CAD build for the part. Positions are in the model's coordinates, mm. A direction names the side the tool comes from. Coordinates: 2 decimals unless noted, no trailing zeros. Write each loop counter-clockwise with the first axis right and the second up, starting at its lowest first coordinate (ties: lowest second). Pieces come first, ordered by that corner, then holes. Notation, with made-up numbers: (-38, 12) - (-18, 12) arc R27 ccw to (-18, 28) - close; hole circle Ø3 at (31.25, 58). An arc over 180 degrees is marked (long way). Answer in a Markdown table with one row per item. Add a question column.
Q1. Two-plate mould, pull along Z, no slides. Class faces 1 (the flat face through (0, -15, 250)), 2 (the cylindrical face through (4.77, -10.61, 51.5)): +Z half, -Z half, draft (parallel to the pull), parting line (faces both ways), or undercut.
Q2. 3-axis set-ups, long thin cutter, end or side, ignore diameter. For faces 3 (the cylindrical face through (-0.96, -4.34, 154.53)), 4 (the cylindrical face through (-0.8, 6.3, 150.3)), 5 (the cylindrical face through (4.77, -10.61, 16.5)): which of +Z, -Z, +X, -X, +Y, -Y reach the whole face in a straight line?
Q3. Band-saw the part on B-B (y = 0). List the corners of the cut face in (x, z) (3 decimals), and give its area (3 significant figures).
Q4. Drill centre lines: line 1 along Z through (x, y) = (-0.25, -7.25); line 2 along Y through (x, z) = (0, 169) (3 decimals); line 3 along Z through (x, y) = (-2.5, -7.5). Where is each one in solid material? Low to high. Write a range as from..to.
Q5. Band-saw the part on C-C (z = 15). List the corners of the cut face in (x, y) (3 decimals), and give its area (3 significant figures).
Q6. Pin check, flat tips, straight feed: pin 1 (6 mm diameter, centred on x = -1.5, z = 69.5, fed in from +Y); pin 2 (3 mm diameter, centred on x = 4, z = 73.5, fed in from -Y); pin 3 (6 mm diameter, centred on x = 1.5, z = 224.5, fed in from -Y); pin 4 (2 mm diameter, centred on x = -5, z = 90.5, fed in from -Y). Stop position of each tip, or through.
Q7. Band-saw the part on D-D (z = 261.5). List the corners of the cut face in (x, y) (3 decimals).
```python
from build123d import *

# Parameters (mm, degrees)
F0_R     = 6.35
F1_DEPTH = 304.8
F2_R     = 5
F4_DEPTH = 15
F3_R     = 4.445
F5_DEPTH = 304.8010001


# Not quite as in the source:
# - a pattern or mirror of a feature is missing from the dataset's text; its kind, count and spacing are read off the source's solid


with BuildPart() as f1:
    # F0 (on Top) → F1 (new body)
    with BuildSketch(Plane.XY):
        Circle(F0_R)
    extrude(amount=F1_DEPTH)

    # F2 (on Front) → F4 (join)
    with BuildSketch(Plane.XZ):
        with Locations((0, 15)):
            Circle(F2_R)
        with Locations((0, 50)):
            Circle(F2_R)
        with Locations((0, 250)):
            Circle(F2_R)
        with Locations((0, 285)):
            Circle(F2_R)
    extrude(amount=F4_DEPTH)

    # F3 (on face) → F5 (cut, through all)
    with BuildSketch(Plane.XY.offset(304.8)):
        Circle(F3_R)
    extrude(amount=-F5_DEPTH, mode=Mode.SUBTRACT)

    # F8: sweep along a path in F6
    with BuildLine(Plane.XY.offset(304.8)) as f8_path:
        CenterArc((0, 0), 5.461, 0, 360)
    # F7 (on Front) → F8 (sweep, cut)
    with BuildSketch(Plane.XZ):
        with BuildLine():
            Line((-5, 304.8), (-6, 304.8))
            ThreePointArc((-6, 304.8), (-5.5, 304.3), (-5, 304.8))
        make_face()
    f8 = sweep(path=f8_path.line, mode=Mode.SUBTRACT)

    # F8_copies: F8 across plane
    add(f8.mirror(Plane(origin=(0, 0, 152.4), x_dir=(-1, 0, 0), z_dir=(0, 0, -1))), mode=Mode.SUBTRACT)


solid = f1.part
```
Checked values:
| question | item | result |
|---|---|---|
| 1 | face 1 | draft |
| 1 | face 2 | undercut |
| 2 | face 3 | +Z, -Z |
| 2 | face 4 | none |
| 2 | face 5 | -Y |
| 3 | outline | (-6.35, 0) - (-6, 0) arc R0.5 cw to (-5, 0) - (-4.445, 0) - (-4.445, 304.8) - (-5, 304.8) arc R0.5 cw to (-6, 304.8) - (-6.35, 304.8) - close; (4.445, 0) - (5, 0) arc R0.5 cw to (6, 0) - (6.35, 0) - (6.35, 304.8) - (6, 304.8) arc R0.5 cw to (5, 304.8) - (4.445, 304.8) - close |
| 3 | area | 1,160 mm² |
| 4 | line 1 | z = 10.01..19.99, 45.01..54.99, 245.01..254.99, 280.01..289.99 |
| 4 | line 2 | y = -6.35..-4.445, 4.445..6.35 |
| 4 | line 3 | z = 10.67..19.33, 45.67..54.33, 245.67..254.33, 280.67..289.33 |
| 5 | outline | (-5, -15) - (5, -15) - (5, -3.914) arc R6.35 ccw (long way) to (-5, -3.914) - close; hole circle Ø8.89 at (0, 0) |
| 5 | area | 158 mm² |
| 6 | pin 1 | stops at y = 6.35 |
| 6 | pin 2 | stops at y = -5.84 |
| 6 | pin 3 | stops at y = -6.35 |
| 6 | pin 4 | stops at y = -4.93 |
| 7 | outline | circle Ø12.7 at (0, 0); hole circle Ø8.89 at (0, 0) |
